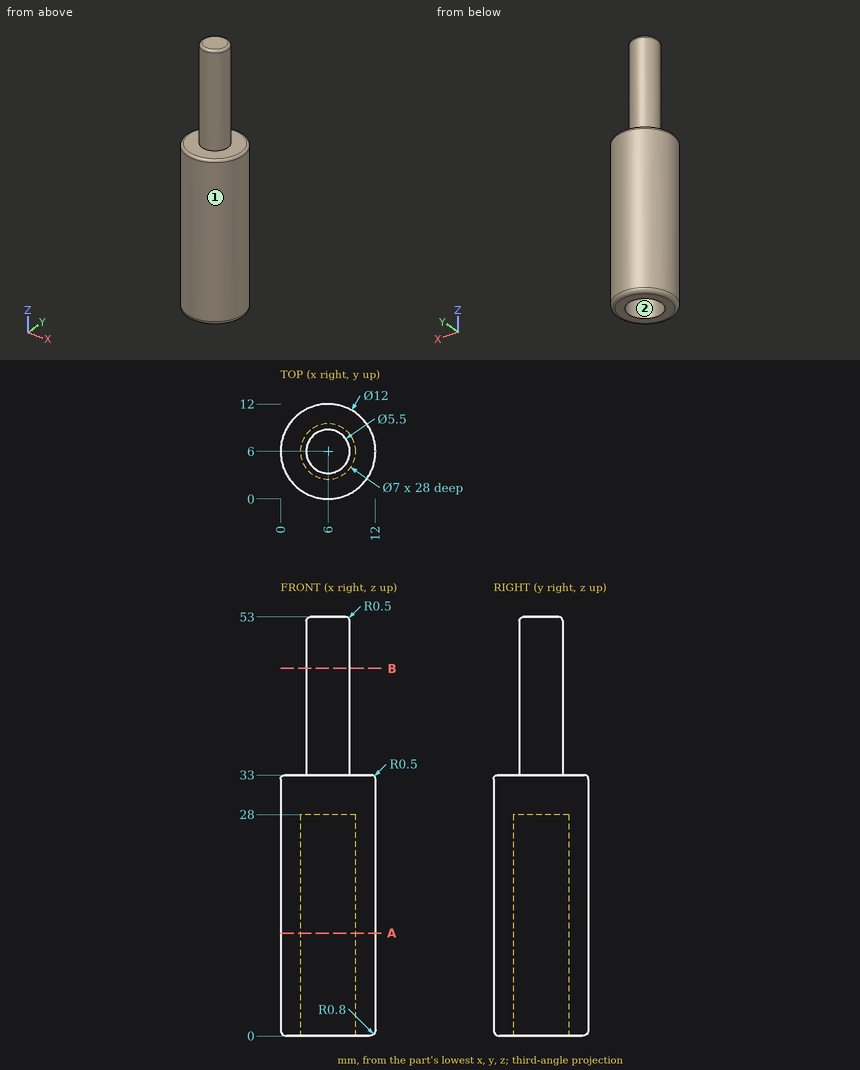
Print and shaded views of the part. All mm, measured from the part's lowest x, y and z. Coordinates: 2 decimals unless noted, no trailing zeros. Loops run counter-clockwise (first coordinate to the right, second up) from the corner with the lowest first, then second, coordinate; pieces in that order, holes last. Notation, with made-up numbers: (-3, 43.5) - (7, 43.5) arc R28 cw to (7, 75.5) - close; hole circle Ø2 at (6.5, 39.5). An arc over 180 degrees is marked (long way). Use one line per item in the form item = value. Start each with the question number.
1) Band-saw the part on A-A (z = 13). Give the cut face in (x, y), and give its area (3 significant figures).
2) Band-saw the part on B-B (z = 46.5). Give the cut face in (x, y).
3) Flat gauge pins, fed straight in: pin 1 (5 mm diameter, centred on x = 10, z = 47.5, fed in from -Y); pin 2 (1 mm diameter, centred on y = 7, z = 13, fed in from +X); pin 3 (4 mm diameter, centred on y = 10, z = 25.5, fed in from -X). Where does each tip first touch, or does it go through?
4) Drill centre lines: L1, parallel to Y at x = 6, z = 4; L2, parallel to Z at x = 6.25, y = 4; L3, parallel to Z at x = 5.5, y = 9.75. Where is each one in solid material? Low to high. Write a range as from..to.
5) Two-plate mould, pull along X, no slides. Class the marked faces 1 and 2: +X half, -X half, draft (parallel to the pull), parting line (faces both ways), or undercut.
Check values:
q1.outline = circle Ø12 at (6, 6); hole circle Ø7 at (6, 6)
q1.area = 74.6 mm2
q2.outline = circle Ø5.5 at (6, 6)
q3.pin_1 = 3.7
q3.pin_2 = 11.98
q3.pin_3 = 0.34
q4.L1 = 0..2.5, 9.5..12
q4.L2 = 28..53
q4.L3 = 0..33
q5.face_1 = parting line
q5.face_2 = undercut
